Work out the finished part from the listing and answer in its coordinate system (mm). A direction names the side the tool comes from. Round coordinates to 2 decimals unless told otherwise and drop trailing zeros. Order: outer loops, then holes, each group sorted by start corner. A loop starts at its lowest first (then second) coordinate and runs counter-clockwise, first axis right, second up. Notation, with made-up numbers: (35, 47.25) -> (82, 47.25) arc R9 cw to (82, 53.25) -> close; hole circle Ø11 at (-38, -8). An arc over 180 degrees is marked (long way). Use one line per item in the form item = value.
```python
from build123d import *

# Parameters (mm, degrees)
F0_R     = 2.5
F1_DEPTH = 6


with BuildPart() as f1:
    # F0 (on Top) → F1 (new body)
    with BuildSketch(Plane.XY):
        Polygon((-46.64715, -20), (-46.64715, -33), (82.85285, -33), (82.85285, -20), (88.85285, -20), (88.85285, -12), (88.85285, -10), (82.85285, -10), (82.85285, 0), (88.85285, 0), (88.85285, 10), (82.85285, 10), (82.85285, 20), (88.85285, 20), (88.85285, 30), (82.85285, 30), (82.85285, 40), (88.85285, 40), (88.85285, 53), (-39.14715, 53), (-39.14715, 40), (-46.64715, 40), (-46.64715, 30), (-40.64715, 30), (-40.64715, 20), (-46.64715, 20), (-46.64715, 10), (-40.64715, 10), (-40.64715, 0), (-46.64715, 0), (-46.64715, -10), (-40.64715, -10), (-40.64715, -20), align=None)
        Polygon((62.60285, 8), (62.60285, 0), (62.60285, -12), (-20.89715, -12), (-20.89715, 0), (-20.89715, 8), align=None, mode=Mode.SUBTRACT)
        with Locations((-9.14715, 22.913525)):
            Circle(F0_R, mode=Mode.SUBTRACT)
        with Locations((-9.14715, 42.913525)):
            Circle(F0_R, mode=Mode.SUBTRACT)
        with Locations((50.85285, 22.913525)):
            Circle(F0_R, mode=Mode.SUBTRACT)
        with Locations((50.85285, 43)):
            Circle(F0_R, mode=Mode.SUBTRACT)
    extrude(amount=F1_DEPTH)


solid = f1.part
```
Item 1: Consider line 1 along Y through (x, z) = (-9, 2.9); line 2 along Y through (x, z) = (-8, 0.65); line 3 along Y through (x, z) = (57, 4.65). Determine where each line is inside the solid, lowest interval first.
Findings:
line_1 = -33 to -12, 8 to 20.42, 25.41 to 40.42, 45.41 to 53
line_2 = -33 to -12, 8 to 20.69, 25.13 to 40.69, 45.13 to 53
line_3 = -33 to -12, 8 to 53
Item 2: Determine the mould class of faces 5 (the flat face through (88.853, 46, 3)), 6 (the flat face through (86, -20, 3)), 7 (the flat face through (-44, 30, 3)) for opening direction Y: released by +Y, released by -Y, zero draft, split by the parting line, or undercut.
Findings:
face_5 = zero draft
face_6 = released by -Y
face_7 = undercut
Item 3: The part is cut by section C-C, the plane y = 16. Give the vertices of the cut face in (x, z).
Findings:
outline = (-46.65, 0) -> (82.85, 0) -> (82.85, 6) -> (-46.65, 6) -> close
Item 4: For faces 1 (the flat face through (20, 11, 6)), 2 (the flat face through (-44, -20, 3)), 3 (the flat face through (62.603, -2, 3)), 4 (the flat face through (86, 10, 3)), determine the directions among +Z, -Z, +X, -X, +Y, -Y from which every point of the face is accessible in a straight line to the end or side of a thin tool.
Findings:
face_1 = +Z, +X, -X, +Y, -Y
face_2 = +Z, -Z, -X
face_3 = +Z, -Z
face_4 = +Z, -Z, +X
Item 5: The part is cut by section D-D, the plane z = 5.1. Give the number of separate pieces and of enclosed holes in the cut face, and give its area (3 significant figures).
Findings:
separate_pieces = 1
enclosed_holes = 5
area = 9,370 mm^2
Item 6: The part is cut by section A-A, the plane x = -14.5. Give the vertices of the cut face in (y, z).
Findings:
outline = (-33, 0) -> (-12, 0) -> (-12, 6) -> (-33, 6) -> close; (8, 0) -> (53, 0) -> (53, 6) -> (8, 6) -> close
Item 7: Flat-ended cylindrical pins translate along their axes: P1, Ø3, axis at x = 86, z = 4.5, coming from the -Y side; P2, Ø3, axis at x = -44.5, z = 3.5, coming from the +Y side; P3, Ø3, axis at y = 34, z = 3, coming from the +X side. Find the tip coordinate at first contact, or state that the pin passes through.
Findings:
P1 = -20
P2 = 40
P3 = 82.85
Item 8: The part is cut by section B-B, the plane y = -1.5. Give the vertices of the cut face in (x, z), and give its area (3 significant figures).
Findings:
outline = (-46.65, 0) -> (-20.9, 0) -> (-20.9, 6) -> (-46.65, 6) -> close; (62.6, 0) -> (82.85, 0) -> (82.85, 6) -> (62.6, 6) -> close
area = 276 mm^2
